Autodesk Inventor part; units mm, degrees
ref_plane "YZ Plane" through (0, 0, 0) normal (1, 0, 0) x (0, 1, 0)
ref_plane "XZ Plane" through (0, 0, 0) normal (0, 1, 0) x (-1, 0, 0)
ref_plane "XY Plane" through (0, 0, 0) normal (0, 0, 1) x (1, 0, 0)
sketch "Sketch1" plane through (0, 0, 0) normal (0, 0, 1) x (1, 0, 0)
  line L0 (0, 0) -> (0, 4368.8557)
  line L1 (0, 4368.8557) -> (100, 4368.8557)
  line L2 (100, 4368.8557) -> (200, 0)
  line L3 (200, 0) -> (0, 0)
  circle A0 centre (0, 0) radius 30
  line L4 (0, 1479.6125) -> (166.1327, 1479.6125)
  line L5 (0, 2959.2249) -> (132.2654, 2959.2249)
  circle A1 centre (0, 1479.6125) radius 30
  circle A2 centre (0, 2959.2249) radius 30
  line L6 (190.7298, 405) -> (120.7298, 405)
  line L7 (120.7298, 405) -> (120.7298, 410)
  line L8 (120.7298, 410) -> (190.7298, 410)
  line L9 (190.7298, 410) -> (190.7298, 405)
  line L10 (109.2882, 909.8691) -> (179.2882, 909.8691)
  line L11 (179.2882, 904.8691) -> (109.2882, 904.8691)
  line L12 (109.2882, 904.8691) -> (109.2882, 909.8691)
  line L13 (179.2882, 909.8691) -> (179.2882, 904.8691)
  line L14 (97.8465, 1409.7381) -> (167.8465, 1409.7381)
  line L15 (167.8465, 1404.7381) -> (97.8465, 1404.7381)
  line L16 (97.8465, 1404.7381) -> (97.8465, 1409.7381)
  line L17 (167.8465, 1409.7381) -> (167.8465, 1404.7381)
  line L18 (86.4049, 1909.6072) -> (156.4049, 1909.6072)
  line L19 (156.4049, 1904.6072) -> (86.4049, 1904.6072)
  line L20 (86.4049, 1904.6072) -> (86.4049, 1909.6072)
  line L21 (156.4049, 1909.6072) -> (156.4049, 1904.6072)
  line L22 (74.9632, 2409.4763) -> (144.9632, 2409.4763)
  line L23 (144.9632, 2404.4763) -> (74.9632, 2404.4763)
  line L24 (74.9632, 2404.4763) -> (74.9632, 2409.4763)
  line L25 (144.9632, 2409.4763) -> (144.9632, 2404.4763)
  line L26 (63.5216, 2909.3454) -> (133.5216, 2909.3454)
  line L27 (133.5216, 2904.3454) -> (63.5216, 2904.3454)
  line L28 (63.5216, 2904.3454) -> (63.5216, 2909.3454)
  line L29 (133.5216, 2909.3454) -> (133.5216, 2904.3454)
  line L30 (52.08, 3409.2144) -> (122.08, 3409.2144)
  line L31 (122.08, 3404.2144) -> (52.08, 3404.2144)
  line L32 (52.08, 3404.2144) -> (52.08, 3409.2144)
  line L33 (122.08, 3409.2144) -> (122.08, 3404.2144)
  line L34 (40.6383, 3909.0835) -> (110.6383, 3909.0835)
  line L35 (110.6383, 3904.0835) -> (40.6383, 3904.0835)
  line L36 (40.6383, 3904.0835) -> (40.6383, 3909.0835)
  line L37 (110.6383, 3909.0835) -> (110.6383, 3904.0835)
  line L38 (0, 1629.6125) -> (162.6993, 1629.6125)
  line L39 (0, 3079.2249) -> (129.5187, 3079.2249)
  point P0 (30, 2959.2249)
  point P1 (0, 2929.2249)
  point P2 (0, 1509.6125)
  point P3 (0, 1449.6125)
  point P4 (0, 30)
  point P5 (30, 0)
  point P6 (190.6154, 410)
  point P7 (179.2882, 904.8691)
  point P8 (179.1737, 909.8691)
  point P9 (167.8465, 1404.7381)
  point P10 (167.7321, 1409.7381)
  point P11 (30, 1479.6125)
  point P12 (156.4049, 1904.6072)
  point P13 (156.2904, 1909.6072)
  point P14 (144.9632, 2404.4763)
  point P15 (144.8488, 2409.4763)
  point P16 (133.5216, 2904.3454)
  point P17 (133.4072, 2909.3454)
  point P18 (0, 2989.2249)
  point P19 (122.08, 3404.2144)
  point P20 (121.9655, 3409.2144)
  point P21 (110.6383, 3904.0835)
  point P22 (110.5239, 3909.0835)
  dimension "d65" = 100
  dimension "d67" = 200
  dimension "d68" = 60
  dimension "d69" = 1480
  dimension "d70" = 1480
  dimension "d71" = 1410
  dimension "d72" = 5
  dimension "d73" = 70
  dimension "d74" = 410
  dimension "d77" = 500
  dimension "d82" = 120
  dimension "d83" = 150
extrude "Plate3" add sketch "Sketch1" along normal blind 4 contours L39 L2 L5 A2 L0 | L0 L1 L2 L34 L36 L35 L30 L32 L31 L39
chamfer "Corner Chamfer2" distance 3 angle 45 4 edges at (122.08, 3404.2144, 2) (121.9655, 3409.2144, 2) (110.6383, 3904.0835, 2) (110.5239, 3909.0835, 2)
equation "\"BendRadius\" = Thickness"
equation "\"BendReliefWidth\" = Thickness"
equation "\"BendReliefDepth\" = 0.5 * Thickness"
equation "\"CornerReliefSize\" = 4 * Thickness"
equation "\"MinimumRemnant\" = 2 * Thickness"
equation "\"TransitionRadius\" = BendRadius"
equation "\"JacobiRadiusSize\" = BendRadius"
equation "\"GapSize\" = Thickness"
properties part number "GBK 3311 central third rib_CPY1" material "Steel"
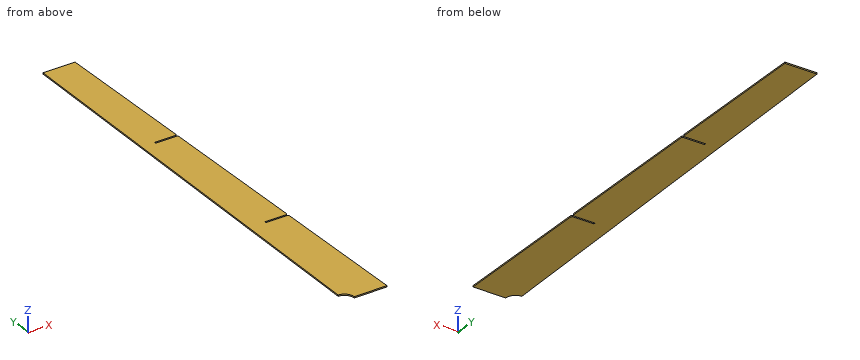
Input: part model. Units: mm. Frame: model coordinates. Round coordinates to 2 decimals unless told otherwise and drop trailing zeros. Loops run counter-clockwise (first coordinate to the right, second up) from the corner with the lowest first, then second, coordinate; pieces in that order, holes last. Notation, with made-up numbers: (-12.75, 26.5) -> (36.25, 26.5) arc R18 ccw to (36.25, 34.5) -> close; hole circle Ø6 at (-6.75, 76.25). An arc over 180 degrees is marked (long way). Use one line per item in the form item = value. Start each with the question number.
Item 1: Section query A-A on z = 2.6. Return the cut outline in (x, y).
Item 2: Section query B-B on y = 3195.5. Return the cut outline in (x, z).
Item 3: Section query C-C on x = 12. Return the cut outline in (y, z), then the cut area to 3 significant figures.
Item 4: Material intervals for L1, parallel to Y at x = 66.5, z = 3.3; L2, parallel to X at y = 4050.5, z = 0.8; L3, parallel to X at y = 3422, z = 2.4, sorted ascending. Write a range as from..to.
Item 5: Contact query for flat-ended pins moving along their axis: pin 1 Ø2 at (y, z) = (3905.5, 1.5) entering from +X; pin 2 Ø1.5 at (x, y) = (30.5, 3920.5) entering from -Z. Output: stop coordinate, or through.
Ans:
q1.outline = (0, 2989.22) arc R30 cw to (30, 2959.22) -> (132.27, 2959.22) -> (122.15, 3401.22) -> (119.08, 3404.21) -> (52.08, 3404.21) -> (52.08, 3409.21) -> (118.97, 3409.21) -> (121.9, 3412.21) -> (110.71, 3901.08) -> (107.64, 3904.08) -> (40.64, 3904.08) -> (40.64, 3909.08) -> (107.52, 3909.08) -> (110.46, 3912.08) -> (100, 4368.86) -> (0, 4368.86) -> close
q2.outline = (0, 0) -> (126.86, 0) -> (126.86, 4) -> (0, 4) -> close
q3.outline = (2986.72, 0) -> (4368.86, 0) -> (4368.86, 4) -> (2986.72, 4) -> close
q3.area = 5,530 mm^2
q4.L1 = 2959.22..3404.21, 3409.21..3904.08, 3909.08..4368.86
q4.L2 = 0..107.29
q4.L3 = 0..121.67
q5.pin_1 = 40.64
q5.pin_2 = 0
